Read the model definition and answer for the solid it produces. Units are mm, in the model's axes. Face numbers are marked on the shaded views. A direction names the side the tool comes from. Round coordinates to 2 decimals unless told otherwise and drop trailing zeros. Write each loop counter-clockwise with the first axis right and the second up, starting at its lowest first coordinate (ties: lowest second). Pieces come first, ordered by that corner, then holes.
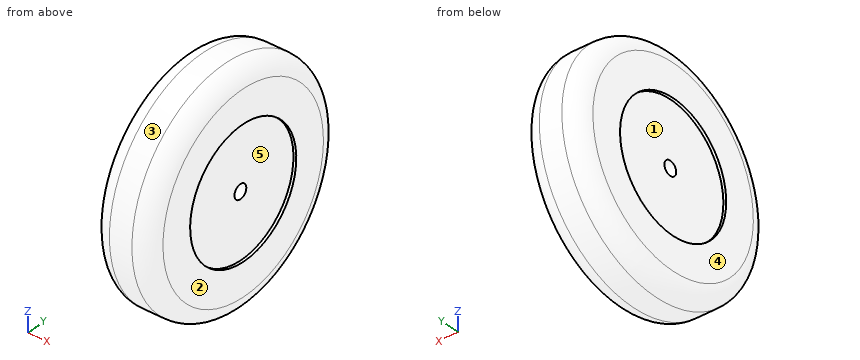
from build123d import *

# Parameters (mm, degrees)
SKETCH1_R           = 50.8
BOSS_EXTRUDE1_DEPTH = 12.7
SKETCH2_R           = 3.175
CUT_EXTRUDE1_DEPTH  = 77.2
FILLET1_R           = 7.62
SKETCH3_R           = 28.575
CUT_EXTRUDE2_DEPTH  = 1.27


with BuildPart() as part:
    # Sketch1 → Boss-Extrude1 (new, symmetric)
    with BuildSketch(Plane(origin=(0, 0, 0), x_dir=(0, 0, -1), z_dir=(1, 0, 0))):
        Circle(SKETCH1_R)
    extrude(amount=BOSS_EXTRUDE1_DEPTH, both=True)

    # Sketch2 → Cut-Extrude1 (cut, through all)
    with BuildSketch(Plane(origin=(12.7, 0, 0), x_dir=(0, 0, -1), z_dir=(1, 0, 0))):
        Circle(SKETCH2_R)
    extrude(amount=-CUT_EXTRUDE1_DEPTH, mode=Mode.SUBTRACT)

    # Fillet1
    fillet1_edges = [part.edges().sort_by_distance(p)[0] for p in [
        (-12.7, 0, 50.8),
        (12.7, 0, 50.8),
    ]]
    fillet(fillet1_edges, radius=FILLET1_R)

    # Sketch3 → Cut-Extrude2 (cut)
    with BuildSketch(Plane(origin=(12.7, 0, 0), x_dir=(0, 0, -1), z_dir=(1, 0, 0))):
        Circle(SKETCH3_R)
    cut_extrude2 = extrude(amount=-CUT_EXTRUDE2_DEPTH, mode=Mode.SUBTRACT)

    # Mirror1: Cut-Extrude2 across plane
    add(cut_extrude2.mirror(Plane(origin=(0, 0, 0), x_dir=(0, 0, 1), z_dir=(1, 0, 0))), mode=Mode.SUBTRACT)


solid = part.part
Q1. Determine the mould class of the marked faces 1, 2 and 3 for opening direction Z: pulls with the +Z half, pulls with the -Z half, needs draft (parallel to the pull), parting line crosses it, or undercut.
Verdict:
face 1: undercut
face 2: needs draft
face 3: parting line crosses it
Q2. Straight lines are drawn through the part: probe 1 along Y at (x, z) = (2, 0) (3 decimals); probe 2 along X at (y, z) = (17.5, 12); probe 3 along Y at (x, z) = (11.9, 0) (3 decimals). For each, find the intervals that lie inside material, in ascending order.
Verdict:
probe 1: y = -50.8 to -3.175, 3.175 to 50.8
probe 2: x = -11.43 to 11.43
probe 3: y = -46.579 to -28.575, 28.575 to 46.579
Q3. Which of the six approach directions +Z, -Z, +X, -X, +Y, -Y give full straight-line access (tool end or side, diameter ignored) to the marked faces 4 and 5?
Verdict:
face 4: +Z, -Z, -X, +Y, -Y
face 5: +X
Q4. Section A-A (y = 0) is taken. Determine the outline of the cut face in (x, z) (3 decimals), then the cut area to 3 significant figures.
Verdict:
outline: (-12.7, -43.18) arc R7.62 ccw to (-5.08, -50.8) - (5.08, -50.8) arc R7.62 ccw to (12.7, -43.18) - (12.7, -28.575) - (11.43, -28.575) - (11.43, -3.175) - (-11.43, -3.175) - (-11.43, -28.575) - (-12.7, -28.575) - close; (-12.7, 28.575) - (-11.43, 28.575) - (-11.43, 3.175) - (11.43, 3.175) - (11.43, 28.575) - (12.7, 28.575) - (12.7, 43.18) arc R7.62 ccw to (5.08, 50.8) - (-5.08, 50.8) arc R7.62 ccw to (-12.7, 43.18) - close
area: 2,240 mm2
Q5. Flat-ended cylindrical pins translate along their axes: pin 1 Ø12 at (x, z) = (-1.5, -1.5) entering from +Y; pin 2 Ø6 at (x, y) = (-6.5, 39) entering from -Z; pin 3 Ø1 at (x, y) = (4.5, -26.5) entering from +Z. Find the tip coordinate at first contact, or state that the pin passes through.
Verdict:
pin 1: stops at y = 50.8
pin 2: stops at z = -35.72
pin 3: stops at z = 43.64
